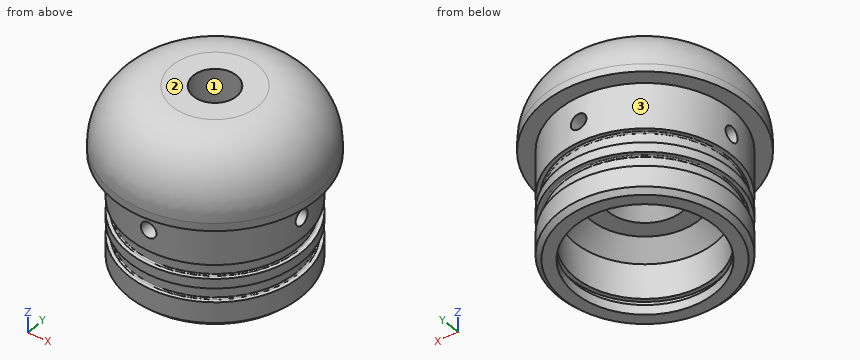
from build123d import *

# Parameters (mm, degrees)
BOSS_EXTRUDE1_START = 2
SKETCH3_R           = 26
SKETCH3_R_2         = 12.25
BOSS_EXTRUDE1_DEPTH = 2
SKETCH11_R          = 12.25
BOSS_EXTRUDE2_DEPTH = 13
SKETCH12_R          = 5.55
CUT_EXTRUDE7_DEPTH  = 28
SKETCH6_R           = 2
CUT_EXTRUDE4_DEPTH  = 6
SKETCH9_R           = 16.5
CUT_EXTRUDE6_DEPTH  = 17.1
CHAMFER1_SIZE       = 4
FILLET1_R           = 0.3
CIRPATTERN1_COUNT   = 4
SKETCH13_R          = 18
CUT_EXTRUDE8_DEPTH  = 17.1
CHAMFER3_SIZE       = 4
SKETCH14_R          = 19
CUT_EXTRUDE9_DEPTH  = 1.6


with BuildPart() as part:
    # Sketch1 → Revolve1 (revolve)
    with BuildSketch(Plane(origin=(0, 0, 0), x_dir=(0, 0, -1), z_dir=(1, 0, 0)), mode=Mode.PRIVATE) as revolve1_sk:
        Polygon((-28.1, 16.231420233), (-28.1, 22.25), (-16.3, 22.25), (-16.3, 21), (-12.7, 21), (-12.7, 22.25), (-10.2, 22.25), (-10.2, 21), (-6.6, 21), (-6.6, 22.25), (-1.2, 22.25), (0, 21.05), (0, 12.25), (-28.1, 12.25), align=None)
    revolve(revolve1_sk.sketch.rotate(Axis((0, 0, 36.316050584), (0, 0, -1)), 180), axis=Axis((0, 0, 36.316050584), (0, 0, -1)))

    # Sketch3 → Boss-Extrude1 (add)
    with BuildSketch(Plane.XY.offset(28.1).offset(BOSS_EXTRUDE1_START)):
        Circle(SKETCH3_R)
        with Locations(Location((0, 0, 0), (0, 0, 270))):
            Circle(SKETCH3_R_2, mode=Mode.SUBTRACT)
    extrude(amount=-BOSS_EXTRUDE1_DEPTH)

    # Sketch4 → Revolve9 (revolve)
    with BuildSketch(Plane(origin=(0, 0, 0), x_dir=(1, 0, 0), z_dir=(0, 1, 0)), mode=Mode.PRIVATE) as revolve9_sk:
        with BuildLine():
            Line((0, -45.1), (0, -30.1))
            Line((0, -30.1), (-26, -30.1))
            ThreePointArc((-26, -30.1), (-21.606601718, -40.706601718), (-11, -45.1))
            Line((-11, -45.1), (0, -45.1))
        make_face()
    revolve(revolve9_sk.sketch.rotate(Axis((0, 0, 0), (0, 0, 1)), 90), axis=Axis((0, 0, 0), (0, 0, 1)))

    # Sketch11 → Boss-Extrude2 (add)
    with BuildSketch(Plane(origin=(0, 0, 30.1), x_dir=(-1, 0, 0), z_dir=(0, 0, -1))):
        with Locations(Location((0, 0, 0), (0, 0, 270))):
            Circle(SKETCH11_R)
    extrude(amount=BOSS_EXTRUDE2_DEPTH)

    # Sketch12 → Cut-Extrude7 (cut)
    with BuildSketch(Plane.XY.offset(45.1)):
        Circle(SKETCH12_R)
    extrude(amount=-CUT_EXTRUDE7_DEPTH, mode=Mode.SUBTRACT)

    # Sketch6 → Cut-Extrude4 (cut)
    with BuildSketch(Plane(origin=(22.25, 0, 0), x_dir=(0, 0, -1), z_dir=(1, 0, 0))):
        with Locations((-21.7, 0)):
            Circle(SKETCH6_R)
    cut_extrude4 = extrude(amount=-CUT_EXTRUDE4_DEPTH, mode=Mode.SUBTRACT)

    # Sketch9 → Cut-Extrude6 (cut)
    with BuildSketch(Plane(origin=(0, 0, 0), x_dir=(-1, 0, 0), z_dir=(0, 0, -1))):
        with Locations(Location((0, 0, 0), (0, 0, 90))):
            Circle(SKETCH9_R)
    extrude(amount=-CUT_EXTRUDE6_DEPTH, mode=Mode.SUBTRACT)

    # Chamfer1
    chamfer1_edges = [part.edges().sort_by_distance(p)[0] for p in [
        (-5.55, 0, 17.1),
        (0, -16.5, 17.1),
    ]]
    chamfer(chamfer1_edges, length=CHAMFER1_SIZE)

    # Fillet1
    fillet1_edges = [part.edges().sort_by_distance(p)[0] for p in [
        (0, 21, 6.6),
        (0, 21, 10.2),
        (0, 21, 12.7),
        (0, 21, 16.3),
    ]]
    fillet(fillet1_edges, radius=FILLET1_R)

    # CirPattern1: Cut-Extrude4 ×4 about axis
    cirpattern1_axis = Axis((0, 0, 0), (0, 0, 1))
    for i in range(1, CIRPATTERN1_COUNT):
        add(cut_extrude4.rotate(cirpattern1_axis, i * 360 / CIRPATTERN1_COUNT), mode=Mode.SUBTRACT)

    # Sketch13 → Cut-Extrude8 (cut)
    with BuildSketch(Plane(origin=(0, 0, 0), x_dir=(-1, 0, 0), z_dir=(0, 0, -1))):
        with Locations(Location((0, 0, 0), (0, 0, 90))):
            Circle(SKETCH13_R)
    extrude(amount=-CUT_EXTRUDE8_DEPTH, mode=Mode.SUBTRACT)

    # Chamfer3
    chamfer3_edges = [part.edges().sort_by_distance(p)[0] for p in [
        (0, -18, 17.1),
    ]]
    chamfer(chamfer3_edges, length=CHAMFER3_SIZE)

    # Sketch14 → Cut-Extrude9 (cut)
    with BuildSketch(Plane(origin=(0, 0, 2.5), x_dir=(-1, 0, 0), z_dir=(0, 0, -1))):
        with Locations(Location((0, 0, 0), (0, 0, 90))):
            Circle(SKETCH14_R)
    extrude(amount=-CUT_EXTRUDE9_DEPTH, mode=Mode.SUBTRACT)


solid = part.part
Design review of the part built by this model. Coordinates are the model's own, in mm. Face numbers are marked on the shaded views. Round coordinates to 2 decimals unless told otherwise and drop trailing zeros. One line per item, written item: value. Start each with the question number.
1) Draft analysis for pull direction X (two halves, no side actions). For the marked faces 1, 2 and 3, state which applies: +X half, -X half, draft (parallel to the pull), parting line (faces both ways), or undercut.
2) To check wall thickness, follow L1, parallel to Y at x = 2, z = 17.5; L2, parallel to X at y = -18.25, z = 21.7; L3, parallel to Z at x = 21, y = -4.5. State the ranges of each line that lie inside material, in increasing order. Write a range as from..to.
3) Insertion check: pin 1 Ø3 at (y, z) = (0.5, 21.5) entering from -X; pin 2 Ø6 at (y, z) = (-9, 32.5) entering from +X; pin 3 Ø1.5 at (x, y) = (-7, -14.5) entering from -Z. Each pin has a flat end and moves straight along its axis. Give the tip position at first contact, or say it passes through.
Reported:
1. face 1: undercut
1. face 2: draft
1. face 3: parting line
2. L1: y = -22.16..-8.93, 8.93..22.16
2. L2: x = -12.73..-2, 2..12.73
2. L3: z = 0.43..6.6, 10.2..12.7, 16.3..40.83
3. pin 1: stops at x = -22.2
3. pin 2: stops at x = 25.19
3. pin 3: stops at z = 14.25
